Read the model definition and answer for the solid it produces. Units are mm, in the model's axes. Face numbers are marked on the shaded views. Give positions to 0.01 mm unless a question says otherwise; leave off trailing zeros. Write each loop counter-clockwise with the first axis right and the second up, starting at its lowest first coordinate (ties: lowest second). Pieces come first, ordered by that corner, then holes. Notation, with made-up numbers: (54.25, 82.5) -> (104.25, 82.5) arc R12 ccw to (104.25, 100.5) -> close; hole circle Ø1 at (-14.75, -7). An arc over 180 degrees is marked (long way). Answer as CSV lines item,"result". Start each with the question number.
1. The part is cut by section A-A, the plane y = 0. Determine the outline of the cut face in (x, z).
2. The part is cut by section D-D, the plane y = 19. Determine the outline of the cut face in (x, z).
3. Given pin 1 (3 mm diameter, centred on x = -21.5, z = 41, fed in from +Y); pin 2 (4 mm diameter, centred on y = 20.5, z = 127.5, fed in from -X); pin 3 (8 mm diameter, centred on y = 0, z = 90, fed in from -X); pin 4 (12 mm diameter, centred on y = -35, z = 21, fed in from -X), each flat-ended and moving along its own axis, determine where each tip first touches the part or whether it passes through.
4. The part is cut by section C-C, the plane z = 90. Determine the outline of the cut face in (x, y).
5. Find the intervals of material crossed by line 1 (Y direction, x = 0, z = 93.5); line 2 (Z direction, x = 45.5, y = 0), in increasing order.
6. The part is cut by section B-B, the plane x = 8.5. Determine the outline of the cut face in (y, z).
7. For a pull along Y with two mould halves and no side action, classify the marked faces 1, 2 and 3 as pulls with the +Y half, pulls with the -Y half, needs draft (parallel to the pull), parting line crosses it, or undercut.
from build123d import *

# Parameters (mm, degrees)
F0_R     = 50
F0_R_2   = 35
F1_DEPTH = 180
F2_R     = 5
F3_DEPTH = 60
F4_COUNT = 6


with BuildPart() as f1:
    # F0 (on Top) → F1 (new body)
    with BuildSketch(Plane.XY):
        Circle(F0_R)
        Circle(F0_R_2, mode=Mode.SUBTRACT)
    extrude(amount=F1_DEPTH)


with BuildPart() as f3:
    # F2 (on Right) → F3 (new body)
    with BuildSketch(Plane.YZ):
        with Locations((0, 90)):
            Circle(F2_R)
    extrude(amount=F3_DEPTH)


with BuildPart() as f4_1:
    # F4: instance of F3
    add(f3.part.rotate(Axis((0, 0, 90), (0, 0, 1)), 1 * 360 / F4_COUNT))


with BuildPart() as f4_2:
    # F4: instance of F3
    add(f3.part.rotate(Axis((0, 0, 90), (0, 0, 1)), 2 * 360 / F4_COUNT))


with BuildPart() as f4_3:
    # F4: instance of F3
    add(f3.part.rotate(Axis((0, 0, 90), (0, 0, 1)), 3 * 360 / F4_COUNT))


with BuildPart() as f4_4:
    # F4: instance of F3
    add(f3.part.rotate(Axis((0, 0, 90), (0, 0, 1)), 4 * 360 / F4_COUNT))


with BuildPart() as f4_5:
    # F4: instance of F3
    add(f3.part.rotate(Axis((0, 0, 90), (0, 0, 1)), 5 * 360 / F4_COUNT))


with BuildPart() as f1_1:
    add(f1.part)

    # F5: cut F4_4, F4_5, F3, F4_1, F4_2, F4_3
    add(f4_4.part, mode=Mode.SUBTRACT)
    add(f4_5.part, mode=Mode.SUBTRACT)
    add(f3.part, mode=Mode.SUBTRACT)
    add(f4_1.part, mode=Mode.SUBTRACT)
    add(f4_2.part, mode=Mode.SUBTRACT)
    add(f4_3.part, mode=Mode.SUBTRACT)


solid = f1_1.part
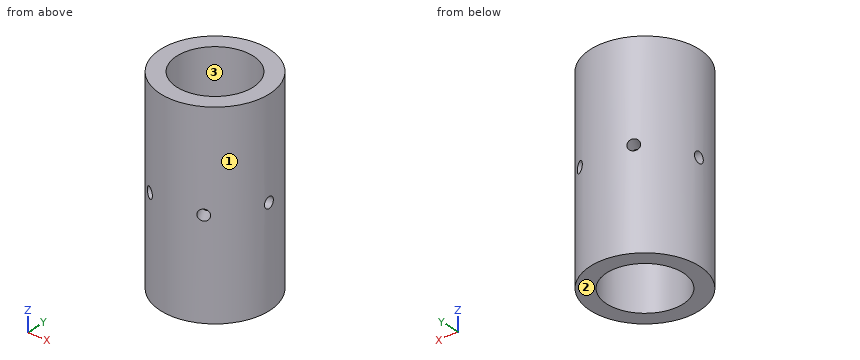
Results found:
1,outline,"(-50, 0) -> (-35, 0) -> (-35, 85) -> (-50, 85) -> close; (-50, 95) -> (-35, 95) -> (-35, 180) -> (-50, 180) -> close; (35, 0) -> (50, 0) -> (50, 85) -> (35, 85) -> close; (35, 95) -> (50, 95) -> (50, 180) -> (35, 180) -> close"
2,outline,"(-46.25, 0) -> (-29.39, 0) -> (-29.39, 180) -> (-46.25, 180) -> close; (29.39, 0) -> (46.25, 0) -> (46.25, 180) -> (29.39, 180) -> close"
3,pin 1,"stops at y = 45.83"
3,pin 2,"stops at x = -46.45"
3,pin 3,"passes through"
3,pin 4,"stops at x = -40.73"
4,outline,"(-49.75, -5) arc R50 ccw to (-29.2, -40.58) -> (-21.65, -27.5) arc R35 cw to (-34.64, -5) -> close; (-49.75, 5) -> (-34.64, 5) arc R35 cw to (-21.65, 27.5) -> (-29.2, 40.58) arc R50 ccw to start; (-20.54, -45.58) arc R50 ccw to (20.54, -45.58) -> (12.99, -32.5) arc R35 cw to (-12.99, -32.5) -> close; (-20.54, 45.58) -> (-12.99, 32.5) arc R35 cw to (12.99, 32.5) -> (20.54, 45.58) arc R50 ccw to start; (21.65, -27.5) -> (29.2, -40.58) arc R50 ccw to (49.75, -5) -> (34.64, -5) arc R35 cw to start; (21.65, 27.5) arc R35 cw to (34.64, 5) -> (49.75, 5) arc R50 ccw to (29.2, 40.58) -> close"
5,line 1,"y = -50 to -35, 35 to 50"
5,line 2,"z = 0 to 85, 95 to 180"
6,outline,"(-49.27, 0) -> (-33.95, 0) -> (-33.95, 180) -> (-49.27, 180) -> close; (33.95, 0) -> (49.27, 0) -> (49.27, 180) -> (33.95, 180) -> close"
7,face 1,"parting line crosses it"
7,face 2,"needs draft"
7,face 3,"undercut"
